Input: part model. Units: mm. Frame: model coordinates. Face numbers are marked on the shaded views. A direction names the side the tool comes from. Coordinates: 2 decimals unless noted, no trailing zeros. Loops run counter-clockwise (first coordinate to the right, second up) from the corner with the lowest first, then second, coordinate; pieces in that order, holes last. Notation, with made-up numbers: M -23,9.5 L 27,9.5 A22 ccw 27,17.5 Z; hole C -38.75,68 d2. An arc over 180 degrees is marked long. Use a Markdown table: item, result. Add a question column.
1. Draft query along Y for the marked faces 3, 4, 5 and 6. Return one class per face: +Y half, -Y half, draft (parallel to the pull), parting line (faces both ways), or undercut.
2. Section A-A on y = 21.5. Output: boundary loops of the cut face in (x, z).
3. Line query: L1, parallel to Y at x = 5.5, z = 6.75; L2, parallel to Y at x = 104.5, z = 9.25; L3, parallel to Y at x = 13, z = 12.75. Output: solid intervals per line, ascending. Write a range as [from, to].
4. Pin query (flat end, axial travel): pin 1 (0.8 mm diameter, centred on x = 5, y = 5, fed in from +Z); pin 2 (0.5 mm diameter, centred on x = 52, z = 0.5, fed in from +Y); pin 3 (3 mm diameter, centred on x = 6, y = 42, fed in from +Z); pin 4 (1 mm diameter, centred on x = 105.5, z = 5, fed in from -Y). Return the tip coordinate at first contact, or that it passes through.
5. Section B-B on x = 17. Output: boundary loops of the cut face in (y, z), then the cut area to 3 significant figures.
6. Set-up query: the marked faces 1 and 2. Return all of +Z, -Z, +X, -X, +Y, -Y with unobstructed straight access to the full face (end or side cutting, diameter ignored); none if empty.
7. Section D-D on z = 6.5. State how many separate pieces and enclosed holes the cut face has, then the cut area to 3 significant figures.
8. Section C-C on x = 57.5. Output: boundary loops of the cut face in (y, z), then the cut area to 3 significant figures.
```python
from build123d import *

# Parameters (mm, degrees)
SKICA1_W                    = 110
SKICA1_H                    = 50
P_IDAT_VYSUNUT_M1_DEPTH     = 13
SKO_EPINA1_T                = -2
SKICA3_W                    = 66.7
SKICA3_H                    = 16
ODEBRAT_VYSUNUT_M1_DEPTH    = 2
SKICA6_R                    = 1.35
SKICA6_W                    = 81.5
SKICA6_H                    = 9.25
P_IDAT_VYSUNUT_M3_DEPTH     = 7.1
SKICA8_W                    = 72
SKICA8_H                    = 27.5
ODEBRAT_VYSUNUT_M2_DEPTH    = 1
ZAOBLIT3_R                  = 1
ZAOBLIT4_R                  = 2
SKICA9_W                    = 81.5
SKICA9_H                    = 6.5
P_IDAT_VYSUNUT_M4_DEPTH     = 1.7
SKICA10_R                   = 1.35
ODEBRAT_VYSUNUT_M3_DEPTH    = 8.8
ZAOBLIT5_R                  = 5
ZAOBLIT6_R                  = 3
SKICA11_R                   = 5
ODEBRAT_VYSUNUT_M4_DEPTH    = 2
ZKOSEN_1_SIZE               = 2
P_IDAT_VYSUNUT_M5_OUTLINE_R = 1.35
P_IDAT_VYSUNUT_M5_DEPTH     = 7.1
SKICA13_W                   = 14.5
SKICA13_H                   = 8
ODEBRAT_VYSUNUT_M5_DEPTH    = 2
ZAOBLIT7_R                  = 1
ZAOBLIT8_R                  = 1
P_IDAT_START                = 1.7
SKICA14_W                   = 6
SKICA14_H                   = 3.5
P_IDAT_VYSUNUT_M6_DEPTH     = 1.7


# Read off the part's stored shape, not the designer's step: Přidat vysunutím5
with BuildPart() as part:
    # Skica1 → Přidat vysunutím1 (new body)
    with BuildSketch(Plane.XY):
        with Locations((55, 25)):
            Rectangle(SKICA1_W, SKICA1_H)
    extrude(amount=P_IDAT_VYSUNUT_M1_DEPTH)

    # Skořepina1
    sko_epina1_openings = [part.faces().sort_by_distance(p)[0] for p in [
        (55, 25, 13),
    ]]
    offset(amount=SKO_EPINA1_T, openings=sko_epina1_openings, kind=Kind.INTERSECTION)

    # Skica3 → Odebrat vysunutím1 (cut)
    with BuildSketch(Plane.XY.offset(2)):
        with Locations((67, 26)):
            Rectangle(SKICA3_W, SKICA3_H)
    extrude(amount=-ODEBRAT_VYSUNUT_M1_DEPTH, mode=Mode.SUBTRACT)

    # Skica6 → Přidat vysunutím3 (add)
    # profile 1 of 3: a face of its own
    with BuildSketch(Plane.XY.offset(2)):
        with BuildLine():
            Line((26.5, 42), (26.5, 48))
            Line((26.5, 48), (32.5, 48))
            Line((32.5, 48), (32.5, 42))
            ThreePointArc((32.5, 42), (29.5, 39), (26.5, 42))
        make_face()
        with Locations((29.5, 42)):
            Circle(SKICA6_R, mode=Mode.SUBTRACT)
    # profile 2 of 3: a face of its own
    with BuildSketch(Plane.XY.offset(2)):
        with BuildLine():
            Line((101.5, 42), (101.5, 48))
            Line((101.5, 48), (108, 48))
            Line((108, 48), (108, 39))
            Line((108, 39), (104.5, 39))
            ThreePointArc((104.5, 39), (102.378679656, 39.878679656), (101.5, 42))
        make_face()
        with Locations((104.5, 42)):
            Circle(SKICA6_R, mode=Mode.SUBTRACT)
    # profile 3 of 3: a face of its own
    with BuildSketch(Plane.XY.offset(2)):
        with Locations((67.25, 6.625)):
            Rectangle(SKICA6_W, SKICA6_H)
    extrude(amount=P_IDAT_VYSUNUT_M3_DEPTH)

    # Skica8 → Odebrat vysunutím2 (cut)
    with BuildSketch(Plane.XY.offset(2)):
        with Locations((67, 26)):
            Rectangle(SKICA8_W, SKICA8_H)
    extrude(amount=-ODEBRAT_VYSUNUT_M2_DEPTH, mode=Mode.SUBTRACT)

    # Zaoblit3
    # the kernel refuses this fillet: 1 mm, written as the material it adds along each edge
    with BuildSketch(Plane(origin=(31, 12.25, 2), x_dir=(1, 0, 0), z_dir=(0, 0, -1)), Plane(origin=(31, 39.75, 2), x_dir=(0, -1, 0), z_dir=(0, 0, -1))) as zaoblit3_piece_1:
        with BuildLine():
            CenterArc((ZAOBLIT3_R, -ZAOBLIT3_R), ZAOBLIT3_R, 90, 90)
            Line((0, -ZAOBLIT3_R), (0, 0))
            Line((0, 0), (ZAOBLIT3_R, 0))
        make_face()
    extrude(amount=1)
    with BuildSketch(Plane(origin=(103, 39.75, 2), x_dir=(0, -1, 0), z_dir=(0, 0, -1)), Plane(origin=(103, 12.25, 2), x_dir=(-1, 0, 0), z_dir=(0, 0, -1))) as zaoblit3_piece_2:
        with BuildLine():
            CenterArc((ZAOBLIT3_R, ZAOBLIT3_R), ZAOBLIT3_R, 180, 90)
            Line((0, ZAOBLIT3_R), (0, 0))
            Line((0, 0), (ZAOBLIT3_R, 0))
        make_face()
    extrude(amount=1)

    # Zaoblit4
    zaoblit4_edges = [part.edges().sort_by_distance(p)[0] for p in [
        (100.35, 18, 0.5),
        (100.35, 34, 0.5),
        (33.65, 34, 0.5),
        (33.65, 18, 0.5),
    ]]
    fillet(zaoblit4_edges, radius=ZAOBLIT4_R)

    # Skica9 → Přidat vysunutím4 (add)
    with BuildSketch(Plane.XY.offset(9.1)):
        with Locations((67.25, 5.25)):
            Rectangle(SKICA9_W, SKICA9_H)
    extrude(amount=P_IDAT_VYSUNUT_M4_DEPTH)

    # Skica10 → Odebrat vysunutím3 (cut)
    with BuildSketch(Plane.XY.offset(10.8)):
        with Locations((104.5, 4.796123071)):
            Circle(SKICA10_R)
        with Locations((29.5, 4.796123071)):
            Circle(SKICA10_R)
    extrude(amount=-ODEBRAT_VYSUNUT_M3_DEPTH, mode=Mode.SUBTRACT)

    # Zaoblit5
    zaoblit5_edges = [part.edges().sort_by_distance(p)[0] for p in [
        (0, 50, 6.5),
        (110, 50, 6.5),
        (110, 0, 6.5),
        (0, 0, 6.5),
    ]]
    fillet(zaoblit5_edges, radius=ZAOBLIT5_R)

    # Zaoblit6
    zaoblit6_edges = [part.edges().sort_by_distance(p)[0] for p in [
        (2, 48, 7.5),
        (2, 2, 7.5),
        (108, 2, 11.9),
        (108, 48, 11.05),
    ]]
    fillet(zaoblit6_edges, radius=ZAOBLIT6_R)

    # Skica11 → Odebrat vysunutím4 (cut)
    with BuildSketch(Plane(origin=(0, 0, 0), x_dir=(-1, 0, 0), z_dir=(0, 0, -1))):
        with Locations((-17, 21.5)):
            Circle(SKICA11_R)
    extrude(amount=-ODEBRAT_VYSUNUT_M4_DEPTH, mode=Mode.SUBTRACT)

    # Zkosení1
    zkosen_1_edges = [part.edges().sort_by_distance(p)[0] for p in [
        (55, 0, 0),
        (0, 25, 0),
        (55, 50, 0),
        (110, 25, 0),
        (1.464466094, 48.535533906, 0),
        (108.535533906, 48.535533906, 0),
        (108.535533906, 1.464466094, 0),
        (1.464466094, 1.464466094, 0),
    ]]
    chamfer(zkosen_1_edges, length=ZKOSEN_1_SIZE)

    # Přidat vysunutím5 outline → Přidat vysunutím5 (add)
    # profile 1 of 2: a face of its own
    with BuildSketch(Plane.XY.offset(2)):
        with BuildLine():
            Line((2, 45), (2, 38.5))
            Line((2, 38.5), (5.5, 38.5))
            ThreePointArc((5.5, 38.5), (7.974873734, 39.525126266), (9, 42))
            Line((9, 42), (9, 48))
            Line((9, 48), (5, 48))
            ThreePointArc((5, 48), (2.878679656, 47.121320344), (2, 45))
        make_face()
        with Locations((5.5, 42)):
            Circle(P_IDAT_VYSUNUT_M5_OUTLINE_R, mode=Mode.SUBTRACT)
    # profile 2 of 2: a face of its own
    with BuildSketch(Plane.XY.offset(2)):
        with BuildLine():
            Line((26.5, 8.5), (2, 8.5))
            Line((2, 8.5), (2, 5))
            ThreePointArc((2, 5), (2.878679656, 2.878679656), (5, 2))
            Line((5, 2), (26.5, 2))
            Line((26.5, 2), (26.5, 8.5))
        make_face()
        with Locations((5.5, 4.796123071)):
            Circle(P_IDAT_VYSUNUT_M5_OUTLINE_R, mode=Mode.SUBTRACT)
    extrude(amount=P_IDAT_VYSUNUT_M5_DEPTH)

    # P_idat vysunut_m5 2 outline → P_idat vysunut_m5 2 (revolve, cut)
    with BuildSketch(Plane(origin=(17, 21.5, 0), x_dir=(1, 0, 0), z_dir=(0, -1, 0))):
        Polygon((5.5, 0), (5, 0.5), (5, 0), align=None)
    revolve(axis=Axis((17, 21.5, 0), (0, 0, 1)), mode=Mode.SUBTRACT)

    # Skica13 → Odebrat vysunutím5 (cut)
    with BuildSketch(Plane.XZ.offset(-48)):
        with Locations((17.25, 6)):
            Rectangle(SKICA13_W, SKICA13_H)
    extrude(amount=-ODEBRAT_VYSUNUT_M5_DEPTH, mode=Mode.SUBTRACT)

    # Zaoblit7
    zaoblit7_edges = [part.edges().sort_by_distance(p)[0] for p in [
        (10, 49, 10),
        (24.5, 49, 10),
    ]]
    fillet(zaoblit7_edges, radius=ZAOBLIT7_R)

    # Zaoblit8
    zaoblit8_edges = [part.edges().sort_by_distance(p)[0] for p in [
        (10, 49, 2),
        (24.5, 49, 2),
    ]]
    fillet(zaoblit8_edges, radius=ZAOBLIT8_R)

    # Skica14 → Přidat vysunutím6 (add)
    with BuildSketch(Plane.XY.offset(9.1).offset(P_IDAT_START)):
        with Locations((29.5, 46.25)):
            Rectangle(SKICA14_W, SKICA14_H)
        with BuildLine():
            Line((101.5, 48), (105, 48))
            ThreePointArc((105, 48), (107.121320344, 47.121320344), (108, 45))
            Line((108, 45), (108, 44.5))
            Line((108, 44.5), (101.5, 44.5))
            Line((101.5, 44.5), (101.5, 48))
        make_face()
    extrude(amount=-P_IDAT_VYSUNUT_M6_DEPTH)


solid = part.part
```
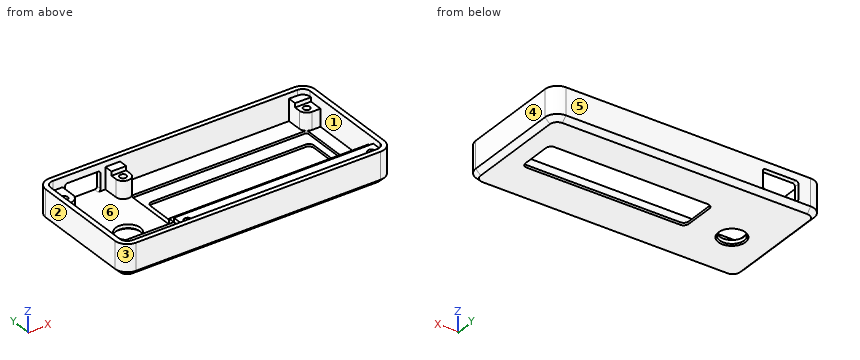
Answers below:
| question | item | result |
|---|---|---|
| 1 | face 3 | -Y half |
| 1 | face 4 | draft |
| 1 | face 5 | +Y half |
| 1 | face 6 | undercut |
| 2 | outline | M 0,2 L 2,0 L 11.5,0 L 12,0.5 L 12,2 L 2,2 L 2,13 L 0,13 Z; M 22,0.5 L 22.5,0 L 33.65,0 L 33.65,1 L 31,1 L 31,2 L 22,2 Z; M 100.35,0 L 108,0 L 110,2 L 110,13 L 108,13 L 108,2 L 103,2 L 103,1 L 100.35,1 Z |
| 3 | L1 | y = [0, 3.45], [6.15, 8.5], [38.5, 40.65], [43.35, 50] |
| 3 | L2 | y = [0, 3.45], [6.15, 8.5], [44.5, 50] |
| 3 | L3 | y = [0, 2], [48, 50] |
| 4 | pin 1 | stops at z = 2 |
| 4 | pin 2 | stops at y = 48.75 |
| 4 | pin 3 | stops at z = 9.1 |
| 4 | pin 4 | stops at y = 0 |
| 5 | outline | M 0,2 L 2,0 L 16,0 L 16.5,0.5 L 16.5,2 L 8.5,2 L 8.5,9.1 L 2,9.1 L 2,13 L 0,13 Z; M 26.5,0.5 L 27,0 L 48,0 L 50,2 L 26.5,2 Z; M 48,10 L 50,10 L 50,13 L 48,13 Z |
| 5 | area | 150 mm² |
| 6 | face 1 | +Z |
| 6 | face 2 | +Z, -Z, -X, +Y, -Y |
| 7 | separate pieces | 1 |
| 7 | enclosed holes | 6 |
| 7 | area | 1,620 mm² |
| 8 | outline | M 0,2 L 2,0 L 18,0 L 18,1 L 12.25,1 L 12.25,2 L 11.25,2 L 11.25,9.1 L 8.5,9.1 L 8.5,10.8 L 2,10.8 L 2,13 L 0,13 Z; M 34,0 L 48,0 L 50,2 L 50,13 L 48,13 L 48,2 L 39.75,2 L 39.75,1 L 34,1 Z |
| 8 | area | 173 mm² |
